from build123d import *

# Parameters (mm, degrees)
CYLINDER_R        = 18
CYLINDER_DEPTH    = 42
SKETCH_R          = 10.2
POCKET_DEPTH      = 16
SKETCH002_R       = 12.5
SKETCH002_R_2     = 3.5
POCKET001_DEPTH   = 18
SKETCH001_R       = 4
POCKET002_DEPTH   = 4
SKETCH003_R       = 1.453406
POCKET003_DEPTH   = 5
CYLINDER001_R     = 1
CYLINDER001_DEPTH = 33
CYLINDER002_R     = 1.5
CYLINDER002_DEPTH = 10
SKETCH004_W       = 3.987101
SKETCH004_H       = 23.792822
POCKET004_DEPTH   = 3


with BuildPart() as part:
    # Cylinder → Cylinder (join)
    with BuildSketch(Plane.XY):
        Circle(CYLINDER_R)
    extrude(amount=CYLINDER_DEPTH)

    # Sketch (on Face2 of Cylinder) → Pocket (cut)
    with BuildSketch(Plane(origin=(0, 0, 0), x_dir=(1, 0, 0), z_dir=(0, 0, -1))):
        with Locations((-7, 0)):
            Circle(SKETCH_R)
    extrude(amount=-POCKET_DEPTH, mode=Mode.SUBTRACT)

    # Sketch002 (on DatumPlane) → Pocket001 (cut)
    with BuildSketch(Plane.XY.offset(42)):
        with Locations((4, 0)):
            Circle(SKETCH002_R)
        with Locations((4, 0)):
            Circle(SKETCH002_R_2, mode=Mode.SUBTRACT)
    extrude(amount=-POCKET001_DEPTH, mode=Mode.SUBTRACT)

    # Sketch001 (on DatumPlane) → Pocket002 (cut)
    with BuildSketch(Plane(origin=(0, 0, 16), x_dir=(1, 0, 0), z_dir=(0, 0, -1))):
        with Locations((-7, 0)):
            Circle(SKETCH001_R)
    extrude(amount=-POCKET002_DEPTH, mode=Mode.SUBTRACT)

    # Sketch003 (on DatumPlane) → Pocket003 (cut)
    with BuildSketch(Plane(origin=(0, 0, 20), x_dir=(1, 0, 0), z_dir=(0, 0, -1))):
        with Locations((-7, 0)):
            Circle(SKETCH003_R)
    extrude(amount=-POCKET003_DEPTH, mode=Mode.SUBTRACT)

    # Cylinder001 → Cylinder001 (cut)
    with BuildSketch(Plane(origin=(-7, 0, 30), x_dir=(0.829038, 0, 0.559193), z_dir=(-0.559193, 0, 0.829038))):
        Circle(CYLINDER001_R)
    extrude(amount=CYLINDER001_DEPTH, mode=Mode.SUBTRACT)

    # Cylinder002 → Cylinder002 (cut)
    with BuildSketch(Plane(origin=(0, 0, 40), x_dir=(0, 1, 0), z_dir=(1, 0, 0))):
        Circle(CYLINDER002_R)
    extrude(amount=CYLINDER002_DEPTH, mode=Mode.SUBTRACT)

    # Sketch004 (on Face2 of Cylinder002) → Pocket004 (cut)
    with BuildSketch(Plane.YX):
        with Locations((0.203517, 6.997041)):
            Rectangle(SKETCH004_W, SKETCH004_H)
    extrude(amount=-POCKET004_DEPTH, mode=Mode.SUBTRACT)


solid = part.part
Work out the finished part from the listing and answer in its coordinate system (mm). A direction names the side the tool comes from. Round coordinates to 2 decimals unless told otherwise and drop trailing zeros. Loops run counter-clockwise (first coordinate to the right, second up) from the corner with the lowest first, then second, coordinate; pieces in that order, holes last. Notation, with made-up numbers: (-14.75, 58.25) - (20.25, 58.25) arc R7 cw to (20.25, 65.25) - close; hole circle Ø1 at (87, -3). An arc over 180 degrees is marked (long way). Use one line per item in the form item = value. Start each with the question number.
(1) Find section D-D on z = 7. Determine the outline of the cut face in (x, y).
(2) Flat-ended cylindrical pins translate along their axes: P1, Ø2, axis at x = -9, z = 26, coming from the -Y side; P2, Ø4.5, axis at x = -7, y = 0, coming from the -Z side; P3, Ø12, axis at x = -7, y = 0, coming from the -Z side. Find the tip coordinate at first contact, or state that the pin passes through.
(3) Find section B-B on z = 28.5. Determine the outline of the cut face in (x, y).
(4) Find section A-A on y = 0. Give the number of separate pieces and of enclosed holes in the cut face, and give its area (3 significant figures).
(5) Determine the mould class of faces 4 (the face through (10, -1.79, 1)), 5 (the face through (3.949, 1.386, 39.425)), 6 (the face through (-2.343, 17.847, 20.706)) for opening direction X: +X half, -X half, draft (parallel to the pull), parting line (faces both ways), or undercut.
(6) Consider line 1 (X direction, y = 0, z = 37.75); line 2 (X direction, y = 0, z = 33); line 3 (X direction, y = 0, z = 18.1). Determine where each line is inside the solid, lowest interval first.
(7) Find section C-C on x = -7. Determine the outline of the cut face in (y, z).
(8) Which of the six approach directions +Z, -Z, +X, -X, +Y, -Y give full straight-line access (tool end or side, diameter ignored) to faces 1 (the face through (7, -3, 24)), 2 (the face through (10, 2.197, 1)), 3 (the face through (-7.1, 4.4, 16))?
Answer list:
q1.outline = circle Ø36 at (0, 0); hole circle Ø20.4 at (-7, 0)
q2.P1 = -16.12
q2.P2 = 20
q2.P3 = 16
q3.outline = circle Ø36 at (0, 0); circle Ø7 at (4, 0); hole circle Ø25 at (4, 0)
q4.separate_pieces = 4
q4.enclosed_holes = 0
q4.area = 729 mm^2
q5.face_4 = draft
q5.face_5 = undercut
q5.face_6 = parting line
q6.line_1 = -18 to -13.43, -11.02 to -8.5, 0.5 to 7.5, 16.5 to 18
q6.line_2 = -18 to -10.23, 0.5 to 7.5, 16.5 to 18
q6.line_3 = -18 to -11, -3 to 18
q7.outline = (-16.58, 0) - (-10.2, 0) - (-10.2, 16) - (-4, 16) - (-4, 20) - (-1.45, 20) - (-1.45, 24) - (-5.94, 24) - (-5.94, 42) - (-16.58, 42) - close; (1.45, 20) - (4, 20) - (4, 16) - (10.2, 16) - (10.2, 0) - (16.58, 0) - (16.58, 42) - (5.94, 42) - (5.94, 24) - (1.45, 24) - close
q8.face_1 = +Z
q8.face_2 = -Z, +X
q8.face_3 = -Z
